Study the drawing (mm; zero at the part's minimum x, y, z) and answer. A direction names the side the tool comes from. Round coordinates to 2 decimals unless told otherwise and drop trailing zeros. Write each loop counter-clockwise with the first axis right and the second up, starting at its lowest first coordinate (ties: lowest second). Pieces come first, ordered by that corner, then holes. Notation, with made-up numbers: (-31, -35.75) - (8, -35.75) arc R14 cw to (8, -21.75) - close; hole circle Ø6 at (18, 0). An arc over 180 degrees is marked (long way). Use one line per item in the form item = value. Start each with the question number.
1) Consider line 1 along Z through (x, y) = (90, 113); line 2 along Y through (x, z) = (53, 42); line 3 along X through (y, z) = (94, 59). Determine where each line is inside the solid, lowest interval first. Write a range as from..to.
2) The part is cut by section C-C, the plane z = 11. Give the vertices of the cut face in (x, y).
3) The part is cut by section B-B, the plane x = 60. Give the vertices of the cut face in (y, z).
4) For the marked faces 1, 2 and 3, determine the directions among +Z, -Z, +X, -X, +Y, -Y from which every point of the face is accessible in a straight line to the end or side of a thin tool.
5) The part is cut by section A-A, the plane y = 4. Give the vertices of the cut face in (x, z).
6) The part is cut by section D-D, the plane y = 79.5. Give the vertices of the cut face in (x, z), plus the area to 3 significant figures.
7) Each of these flat-tipped pins is pushed along its axis until it touches: pin 1 (6 mm diameter, centred on x = 58.5, z = 19.5, fed in from -Y); pin 2 (24.5 mm diameter, centred on y = 13, z = 43.5, fed in from -X); pin 3 (4 mm diameter, centred on x = 80, y = 110, fed in from -Z); pin 4 (2.5 mm diameter, centred on x = 50.28, y = 4, fed in from +Z). Where does it stop, or does it pass through?
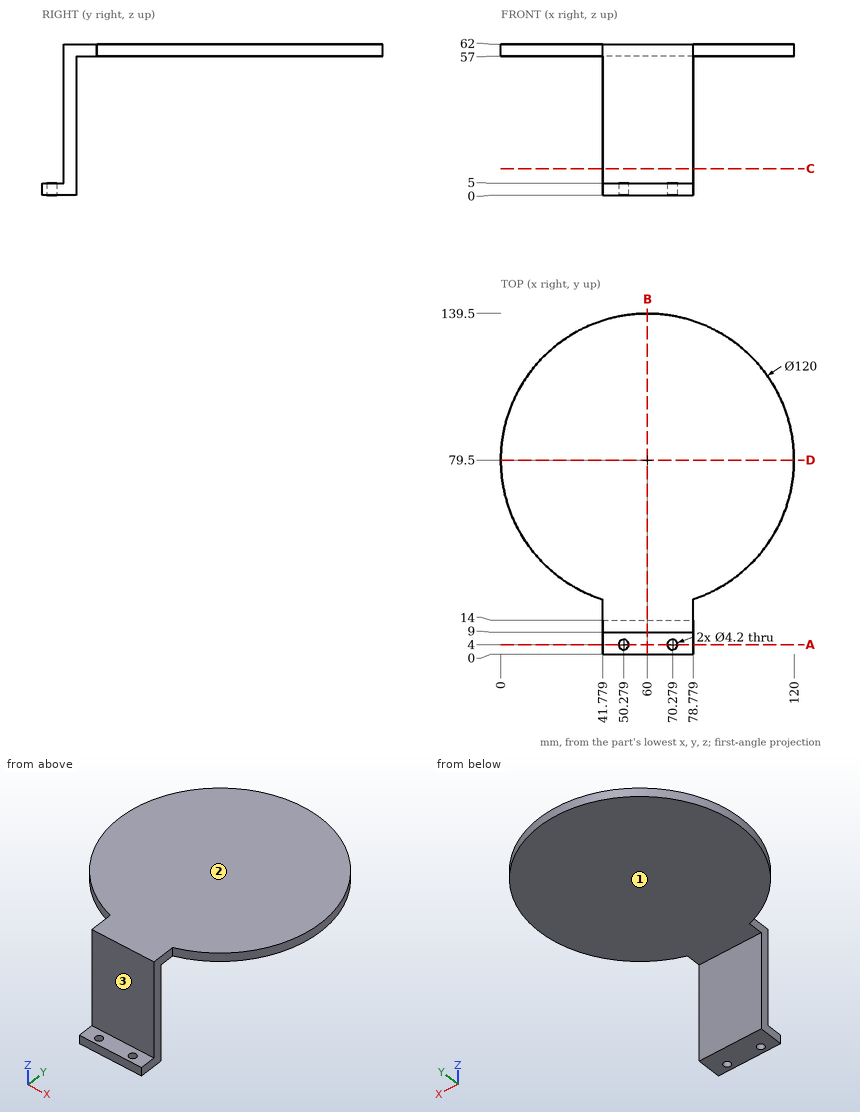
Geometry results:
q1.line_1 = 57..62
q1.line_2 = 9..14
q1.line_3 = 1.78..118.22
q2.outline = (41.78, 9) - (78.78, 9) - (78.78, 14) - (41.78, 14) - close
q3.outline = (0, 0) - (14, 0) - (14, 57) - (139.5, 57) - (139.5, 62) - (9, 62) - (9, 5) - (0, 5) - close
q4.face_1 = -Z, +X, -X, +Y
q4.face_2 = +Z, +X, -X, +Y, -Y
q4.face_3 = +Z, +X, -X, -Y
q5.outline = (41.78, 0) - (48.18, 0) - (48.18, 5) - (41.78, 5) - close; (52.38, 0) - (68.18, 0) - (68.18, 5) - (52.38, 5) - close; (72.38, 0) - (78.78, 0) - (78.78, 5) - (72.38, 5) - close
q6.outline = (0, 57) - (120, 57) - (120, 62) - (0, 62) - close
q6.area = 600 mm2
q7.pin_1 = 9
q7.pin_2 = 41.78
q7.pin_3 = 57
q7.pin_4 = through
